Here's how the part is built. I have some questions about the finished solid (model axes, mm). A direction names the side the tool comes from. Give positions to 0.01 mm unless a question says otherwise; leave off trailing zeros. Use CSV: the item, a comma, the result in double quotes. Start each with the question number.
(1) Which directions (+Z, -Z, +X, -X, +Y, -Y) give clear straight access to the entire face, cutting with the end or side of a thin tool? Please do faces 1 (the flat face through (203, 13, -25.4)), 2 (the flat face through (203, 13, -3.175)).
(2) I need wall thicknesses on L1, parallel to Y at x = 347, z = -9 (3 decimals); L2, parallel to Z at x = 189, y = 4.25 (3 decimals); L3, parallel to X at y = 1.85, z = -12.7. Which ranges of each line are inside material? Lowest first, please. Write a range as [from, to].
(3) If we mould it in two halves opening along Y, with no side actions, what happens to faces 3 (the flat face through (203, 25.4, -13)), 4 (the flat face through (197, 22.225, -13)), 5 (the flat face through (203, 0, -13))? For each: pulls with the +Y half, pulls with the -Y half, needs draft (parallel to the pull), parting line crosses it, or undercut.
Autodesk Inventor part; units mm, degrees
ref_plane "Work Plane1" through (200.025, 0, 0) normal (1, 0, 0) x (0, 0, -1)
ref_plane "YZ Plane" through (0, 0, 0) normal (1, 0, 0) x (0, 1, 0)
ref_plane "XZ Plane" through (0, 0, 0) normal (0, 1, 0) x (-1, 0, 0)
sketch "Sketch1" plane through (0, 0, 0) normal (0, 1, 0) x (-1, 0, 0)
  line L0 (0, 0) -> (-400.05, 0)
  line L1 (-400.05, 0) -> (-400.05, -25.4)
  line L2 (-400.05, -25.4) -> (0, -25.4)
  line L3 (0, -25.4) -> (0, 0)
  dimension "d0" = 400.05
  dimension "d1" = 25.4
extrude "Extrusion1" add sketch "Sketch1" along normal blind 3.175
ref_plane "Work Plane1" through (200.025, 0, 0) normal (1, 0, 0) x (0, 0, -1)
sketch "Sketch7" plane through (0, 3.175, 0) normal (0, 1, 0) x (1, 0, 0)
  line L0 (400.05, 0) -> (400.05, 25.4)
  line L1 (0, 0) -> (400.05, 0)
  line L2 (400.05, 0) -> (400.05, 3.175)
  line L3 (400.05, 3.175) -> (0, 3.175)
  line L4 (0, 3.175) -> (0, 0)
  dimension "d49" = 3.175
extrude "Extrusion2" add sketch "Sketch7" along normal blind 22.225
ref_plane "Work Plane2" through (0, 0, -12.7) normal (0, 0, 1) x (1, 0, 0)
mirror "Mirror2" about plane through (0, 0, -12.7) normal (0, 0, 1) of "Extrusion2"
sketch "Sketch8" plane through (0, 3.175, -22.225) normal (0, 0, 1) x (1, 0, 0)
  line L0 (400.05, 22.225) -> (0, 22.225)
  line L1 (400.05, 22.225) -> (0, 22.225)
  line L2 (0, 22.225) -> (0, 19.05)
  line L3 (0, 19.05) -> (400.05, 19.05)
  line L4 (400.05, 19.05) -> (400.05, 22.225)
  point P0 (0, -3.175)
  dimension "d52" = 400.05
  dimension "d53" = 3.175
extrude "Extrusion3" add sketch "Sketch8" along normal blind 19.05
ref_plane "Work Plane3" through (0, 12.7, 0) normal (0, -1, 0) x (1, 0, 0)
sketch "Sketch10" plane through (400.05, 0, -25.4) normal (0, 0, -1) x (-1, 0, 0)
  line L0 (0, 0) -> (400.05, 0)
  line L1 (0, 0) -> (0, 25.4)
  point P0 (59.0956, 10.1854)
  dimension "d61" = 10.1854
  dimension "d62" = 59.0956
sketch "Sketch11" plane through (400.05, 0, -25.4) normal (0, 0, -1) x (-1, 0, 0)
  line L0 (0, 0) -> (400.05, 0)
  line L1 (0, 0) -> (0, 25.4)
  point P0 (33.6956, 10.1854)
  dimension "d70" = 10.1854
  dimension "d71" = 33.6956
hole "Hole8" at (340.9544, 10.1854, -25.4) direction (0, 0, 1) diameter 5.1594 end through all
hole "Hole9" at (366.3544, 10.1854, -25.4) direction (0, 0, 1) diameter 5.1594 end through all
sketch "Sketch14" plane through (0, 0, 0) normal (0, -1, 0) x (1, 0, 0)
  line L0 (400.05, 0) -> (400.05, -25.4)
  line L1 (400.05, -25.4) -> (0, -25.4)
  point P0 (0, 0)
  point P1 (353.6442, -12.7)
  dimension "d97" = 46.4058
  dimension "d98" = 12.7
hole "Hole10" at (353.6442, 0, -12.7) direction (0, 1, 0) diameter 6.35 end through all
equation "\"d84\" = Thickness"
equation "\"d91\" = Thickness"
equation "\"d104\" = Thickness"
equation "\"BendRadius\" = Thickness"
equation "\"BendReliefWidth\" = Thickness"
equation "\"BendReliefDepth\" = 0.5 * Thickness"
equation "\"CornerReliefSize\" = 4 * Thickness"
equation "\"MinimumRemnant\" = 2 * Thickness"
equation "\"TransitionRadius\" = BendRadius"
equation "\"JacobiRadiusSize\" = BendRadius"
equation "\"GapSize\" = Thickness"
properties part number "Large crossbeam" material "Aluminum 6061"
Geometry says:
1,face 1,"-Z, +X, -X, +Y, -Y"
1,face 2,"+X, -X"
2,L1,"[0, 3.175], [22.225, 25.4]"
2,L2,"[-25.4, -22.225], [-3.175, 0]"
2,L3,"[0, 350.47], [356.82, 400.05]"
3,face 3,"pulls with the +Y half"
3,face 4,"undercut"
3,face 5,"pulls with the -Y half"
